from build123d import *

# Parameters (mm, degrees)
BOSS_EXTRUDE2_DEPTH = 150
SKETCH3_W           = 100
SKETCH3_H           = 280
CUT_EXTRUDE3_DEPTH  = 260.615099715
FILLET2_START       = -151
FILLET2_DEPTH       = 302
FILLET2_START_2     = -150
FILLET2_2_DEPTH     = 100
FILLET2_START_3     = 50
FILLET2_3_DEPTH     = 100
FILLET3_R           = 5


with BuildPart() as part:
    # Sketch2 → Boss-Extrude2 (new, symmetric)
    with BuildSketch(Plane(origin=(0, 0, 0), x_dir=(0, 0, -1), z_dir=(1, 0, 0))):
        Polygon((-60, 10), (-10, 10), (-10, 200), (0, 200), (0, 0), (-26, 0), (-70, 0), (-70, 40), (-60, 40), align=None)
    extrude(amount=BOSS_EXTRUDE2_DEPTH, both=True)

    # Sketch3 → Cut-Extrude3 (cut, through all)
    with BuildSketch(Plane.XY.offset(70)):
        Rectangle(SKETCH3_W, SKETCH3_H)
    extrude(amount=-CUT_EXTRUDE3_DEPTH, mode=Mode.SUBTRACT)

    # Fillet2: read off the stored shape, not the designer's step
    # Fillet2 outline → Fillet2 (cut)
    with BuildSketch(Plane.YZ.offset(FILLET2_START)):
        with BuildLine():
            Line((0, 0), (10, 0))
            ThreePointArc((10, 0), (2.928932188, 2.928932188), (0, 10))
            Line((0, 10), (0, 0))
        make_face()
        with BuildLine():
            Line((0, 70), (0, 60))
            ThreePointArc((0, 60), (2.928932188, 67.071067812), (10, 70))
            Line((10, 70), (0, 70))
        make_face()
    extrude(amount=FILLET2_DEPTH, mode=Mode.SUBTRACT)

    # Fillet2 2 outline → Fillet2 2 (add)
    with BuildSketch(Plane.YZ.offset(FILLET2_START_2)):
        with BuildLine():
            Line((10, 60), (10, 50))
            ThreePointArc((10, 50), (12.928932188, 57.071067812), (20, 60))
            Line((20, 60), (10, 60))
        make_face()
        with BuildLine():
            ThreePointArc((20, 10), (12.928932188, 12.928932188), (10, 20))
            Line((10, 20), (10, 10))
            Line((10, 10), (20, 10))
        make_face()
    extrude(amount=FILLET2_2_DEPTH)

    # Fillet2 3 outline → Fillet2 3 (add)
    with BuildSketch(Plane.YZ.offset(FILLET2_START_3)):
        with BuildLine():
            Line((10, 60), (10, 50))
            ThreePointArc((10, 50), (12.928932188, 57.071067812), (20, 60))
            Line((20, 60), (10, 60))
        make_face()
        with BuildLine():
            ThreePointArc((20, 10), (12.928932188, 12.928932188), (10, 20))
            Line((10, 20), (10, 10))
            Line((10, 10), (20, 10))
        make_face()
    extrude(amount=FILLET2_3_DEPTH)

    # Fillet3
    fillet3_edges = [part.edges().sort_by_distance(p)[0] for p in [
        (0, 200, 10),
    ]]
    fillet(fillet3_edges, radius=FILLET3_R)


solid = part.part
Check sheet for the modelled part. Datum: model origin and axes. Units: mm. A direction names the side the tool comes from. Round coordinates to 2 decimals unless told otherwise and drop trailing zeros. Order: outer loops, then holes, each group sorted by start corner. A loop starts at its lowest first (then second) coordinate and runs counter-clockwise, first axis right, second up.
(1) Draft check along Z on faces 1 (the flat face through (101, 30, 60)), 2 (the flat face through (2, 149, 0)), 3 (the flat face through (101, 40, 65)). Enter one of: pulls with the +Z half, pulls with the -Z half, needs draft (parallel to the pull), parting line crosses it, or undercut.
(2) Cross-section at D-D, the plane x = 60. Enter the section's corners in (y, z).
(3) Go/stop test with flat-tipped pins: P1, Ø6, axis at x = -97, z = 45.5, coming from the -Y side; P2, Ø2, axis at x = 43, y = 153, coming from the +Z side; P3, Ø9, axis at x = 89, z = 31, coming from the +Y side; P4, Ø3, axis at x = 81.5, z = 63, coming from the -Y side. Record where each tip stops, or that it passes through.
(4) Cross-section at A-A, the plane y = 29. Enter the section's corners in (x, z), and give its area (3 significant figures).
(5) Cross-section at B-B, the plane z = 26.5. Enter the section's corners in (x, y).
(6) Access from +Z, -Z, +X, -X, +Y, -Y to the whole of each face (thin tool, end or side, straight path). Record for faces 4 (the flat face through (-99, 40, 65)), 5 (the cylindrical face through (99.3, 2.85, 66.99)), 6 (the flat face through (50, 49, 9)), 7 (the flat face through (-99, 30, 60)).
(7) Scan lines: probe 1 along Z at (x, y) = (87.5, 72.5); probe 2 along Z at (x, y) = (134, 26); probe 3 along Z at (x, y) = (-92, 13). Record each from-to range of solid material in increasing order.
Check sheet entries:
1. face 1: undercut
1. face 2: pulls with the -Z half
1. face 3: needs draft
2. outline: (0, 10) arc R10 ccw to (10, 0) - (200, 0) - (200, 5) arc R5 ccw to (195, 10) - (20, 10) arc R10 cw to (10, 20) - (10, 50) arc R10 cw to (20, 60) - (40, 60) - (40, 70) - (10, 70) arc R10 ccw to (0, 60) - close
3. P1: stops at y = 0
3. P2: stops at z = 10
3. P3: stops at y = 10
3. P4: stops at y = 0.11
4. outline: (-150, 0) - (-50, 0) - (-50, 10) - (-150, 10) - close; (-150, 60) - (-50, 60) - (-50, 70) - (-150, 70) - close; (50, 0) - (150, 0) - (150, 10) - (50, 10) - close; (50, 60) - (150, 60) - (150, 70) - (50, 70) - close
4. area: 4,000 mm2
5. outline: (-150, 0) - (-50, 0) - (-50, 10) - (-150, 10) - close; (50, 0) - (150, 0) - (150, 10) - (50, 10) - close
6. face 4: +Z, +X, -X, +Y
6. face 5: +Z, +X, -X, -Y
6. face 6: +Z, -Z, -Y
6. face 7: +X, -X, +Y
7. probe 1: z = 0 to 10
7. probe 2: z = 0 to 10, 60 to 70
7. probe 3: z = 0 to 12.86, 57.14 to 70
